Check sheet for the modelled part. Datum: model origin and axes. Units: mm. A direction names the side the tool comes from. Round coordinates to 2 decimals unless told otherwise and drop trailing zeros. Loops run counter-clockwise (first coordinate to the right, second up) from the corner with the lowest first, then second, coordinate; pieces in that order, holes last. Notation, with made-up numbers: (17.25, 86.5) -> (54.25, 86.5) arc R27 ccw to (54.25, 113.5) -> close; hole circle Ø11 at (-13.75, 9.5). An arc over 180 degrees is marked (long way). One line per question, with ' | ' between items.
```python
from build123d import *

# Parameters (mm, degrees)
SKETCH1_W           = 200
SKETCH1_H           = 150
BOSS_EXTRUDE1_DEPTH = 3
BOSS_EXTRUDE2_DEPTH = 20
SKETCH3_W           = 10
SKETCH3_H           = 10
BOSS_EXTRUDE3_DEPTH = 3
SKETCH4_W           = 10
SKETCH4_H           = 10
CUT_EXTRUDE1_DEPTH  = 127.589889012
SKETCH5_W           = 10
SKETCH5_H           = 10
BOSS_EXTRUDE4_DEPTH = 3
SKETCH6_W           = 10
SKETCH6_H           = 10
CUT_EXTRUDE2_DEPTH  = 3
SKETCH7_R           = 1.5
CUT_EXTRUDE3_DEPTH  = 127.589889012
SKETCH8_R           = 1.5
CUT_EXTRUDE4_DEPTH  = 127.589889012
SKETCH10_W          = 18
SKETCH10_H          = 13
CUT_EXTRUDE5_DEPTH  = 3


with BuildPart() as part:
    # Sketch1 → Boss-Extrude1 (new body)
    with BuildSketch(Plane(origin=(0, 0, 0), x_dir=(1, 0, 0), z_dir=(0, 1, 0))):
        Rectangle(SKETCH1_W, SKETCH1_H)
    extrude(amount=BOSS_EXTRUDE1_DEPTH)

    # Sketch2 → Boss-Extrude2 (add)
    with BuildSketch(Plane(origin=(0, 3, 0), x_dir=(1, 0, 0), z_dir=(0, 1, 0))):
        Polygon((100, -5), (90, -5), (90, 5), (100, 5), (100, 75), (-100, 75), (-100, 5), (-90, 5), (-90, -5), (-100, -5), (-100, -75), (100, -75), align=None)
        Polygon((97, -8), (87, -8), (87, 8), (97, 8), (97, 72), (-97, 72), (-97, 8), (-87, 8), (-87, -8), (-97, -8), (-97, -72), (97, -72), align=None, mode=Mode.SUBTRACT)
    extrude(amount=BOSS_EXTRUDE2_DEPTH)

    # Sketch3 → Boss-Extrude3 (add)
    with BuildSketch(Plane(origin=(0, 23, 0), x_dir=(1, 0, 0), z_dir=(0, 1, 0))):
        with Locations((-95, 0)):
            Rectangle(SKETCH3_W, SKETCH3_H)
    extrude(amount=-BOSS_EXTRUDE3_DEPTH)

    # Sketch4 → Cut-Extrude1 (cut, through all)
    with BuildSketch(Plane(origin=(0, 3, 0), x_dir=(1, 0, 0), z_dir=(0, 1, 0))):
        with Locations((-95, 0)):
            Rectangle(SKETCH4_W, SKETCH4_H)
    extrude(amount=-CUT_EXTRUDE1_DEPTH, mode=Mode.SUBTRACT)

    # Sketch5 → Boss-Extrude4 (add)
    with BuildSketch(Plane(origin=(0, 23, 0), x_dir=(1, 0, 0), z_dir=(0, 1, 0))):
        with Locations((95, 0)):
            Rectangle(SKETCH5_W, SKETCH5_H)
    extrude(amount=-BOSS_EXTRUDE4_DEPTH)

    # Sketch6 → Cut-Extrude2 (cut)
    with BuildSketch(Plane(origin=(0, 3, 0), x_dir=(1, 0, 0), z_dir=(0, 1, 0))):
        with Locations((95, 0)):
            Rectangle(SKETCH6_W, SKETCH6_H)
    extrude(amount=-CUT_EXTRUDE2_DEPTH, mode=Mode.SUBTRACT)

    # Sketch7 → Cut-Extrude3 (cut, through all)
    with BuildSketch(Plane.XZ.offset(-20)):
        with Locations(Location((95, 0, 0), (0, 0, 270))):
            Circle(SKETCH7_R)
    extrude(amount=-CUT_EXTRUDE3_DEPTH, mode=Mode.SUBTRACT)

    # Sketch8 → Cut-Extrude4 (cut, through all)
    with BuildSketch(Plane.XZ.offset(-20)):
        with Locations(Location((-94.5, 0, 0), (0, 0, 270))):
            Circle(SKETCH8_R)
    extrude(amount=-CUT_EXTRUDE4_DEPTH, mode=Mode.SUBTRACT)

    # Sketch10 → Cut-Extrude5 (cut)
    with BuildSketch(Plane.XY.offset(75)):
        with Locations((0, 16.5)):
            Rectangle(SKETCH10_W, SKETCH10_H)
    extrude(amount=-CUT_EXTRUDE5_DEPTH, mode=Mode.SUBTRACT)


solid = part.part
```
(1) Sectioned sample at A-A, the plane y = 7.75. Record the cut outline in (x, z), and give its area (3 significant figures).
Answer:
outline: (-100, -75) -> (100, -75) -> (100, -5) -> (90, -5) -> (90, 5) -> (100, 5) -> (100, 75) -> (-100, 75) -> (-100, 5) -> (-90, 5) -> (-90, -5) -> (-100, -5) -> close; hole (-97, -72) -> (97, -72) -> (97, -8) -> (87, -8) -> (87, 8) -> (97, 8) -> (97, 72) -> (-97, 72) -> (-97, 8) -> (-87, 8) -> (-87, -8) -> (-97, -8) -> close | area: 2,180 mm2
(2) Set-up check for faces 1 (the face through (93.8, 20, -1.2)), 2 (the face through (1, 13, -72)), 3 (the face through (-96.2, 20, -0.1)): record each of +Z, -Z, +X, -X, +Y, -Y from which the full face is reachable in a straight line by a thin tool's end or side.
Answer:
face 1: +X, -Y | face 2: +Y | face 3: -X, -Y
(3) Scan lines: probe 1 along Z at (x, y) = (-94.5, 21.55); probe 2 along X at (y, z) = (20.8, 0); probe 3 along X at (y, z) = (16.25, 3). Record each from-to range of solid material in increasing order.
Answer:
probe 1: z = -75 to -72, -8 to -1.5, 1.5 to 8, 72 to 75 | probe 2: x = -100 to -96, -93 to -87, 87 to 93.5, 96.5 to 100 | probe 3: x = -90 to -87, 87 to 90
(4) Go/stop test with flat-tipped pins: pin 1 (1.5 mm diameter, centred on y = 13.5, z = -1, fed in from -X); pin 2 (11 mm diameter, centred on y = 15, z = 1, fed in from -X); pin 3 (4 mm diameter, centred on x = 95, z = 0, fed in from -Y); pin 4 (0.9 mm diameter, centred on x = -1.5, z = 74, fed in from +Y). Record where each tip stops, or that it passes through.
Answer:
pin 1: stops at x = -90 | pin 2: stops at x = -100 | pin 3: stops at y = 20 | pin 4: stops at y = 10
(5) Sectioned sample at C-C, the plane x = -28.5. Record the cut outline in (y, z).
Answer:
outline: (0, -75) -> (23, -75) -> (23, -72) -> (3, -72) -> (3, 72) -> (23, 72) -> (23, 75) -> (0, 75) -> close
(6) Sectioned sample at B-B, the plane z = -44.5. Record the cut outline in (x, y).
Answer:
outline: (-100, 0) -> (100, 0) -> (100, 23) -> (97, 23) -> (97, 3) -> (-97, 3) -> (-97, 23) -> (-100, 23) -> close
(7) Mould release check, pull along X, two halves, no side actions. Record for faces 4 (the face through (95, 10, 5)), 5 (the face through (-90, 10, 0)), 6 (the face through (-87, 13, 0)): +X half, -X half, draft (parallel to the pull), parting line (faces both ways), or undercut.
Answer:
face 4: draft | face 5: -X half | face 6: undercut
